Work out the finished part from the listing and answer in its coordinate system (mm). A direction names the side the tool comes from. Round coordinates to 2 decimals unless told otherwise and drop trailing zeros. Order: outer loops, then holes, each group sorted by start corner. A loop starts at its lowest first (then second) coordinate and runs counter-clockwise, first axis right, second up. Notation, with made-up numbers: (13.5, 86.5) - (29.5, 86.5) arc R13 ccw to (29.5, 100.5) - close; hole circle Ø7 at (-35, 75.25). An arc over 180 degrees is marked (long way). Put each result on its own line as item: value.
Autodesk Inventor part; units mm, degrees
ref_plane "YZ Plane" through (0, 0, 0) normal (1, 0, 0) x (0, 1, 0)
ref_plane "XZ Plane" through (0, 0, 0) normal (0, 1, 0) x (-1, 0, 0)
ref_plane "XY Plane" through (0, 0, 0) normal (0, 0, 1) x (1, 0, 0)
sketch "Esboço1" plane through (0, 0, 0) normal (0, 0, 1) x (1, 0, 0)
  line L0 (0, 0) -> (10, 0)
  line L1 (0, 51.1555) -> (0, 0)
  line L2 (2, 35) -> (2, 18.8445)
  line L3 (2, 35) -> (2, 51.1555)
  arc A0 (2, 18.8445) -> (10, 0) centre (66.25, 35) ccw
  line L4 (2, 51.1555) -> (0, 51.1555)
extrude "Extrusão1" add sketch "Esboço1" along normal blind 80
sketch "Esboço2" plane through (0, 0, 80) normal (0, 0, 1) x (1, 0, 0)
  line L0 (0, 0) -> (10, 0)
  line L1 (0, 0) -> (-3, 0)
  line L2 (-5, 2) -> (-5, 2.6)
  line L3 (-5, 2.6) -> (0, 2.6)
  line L4 (-3, 0) -> (-5, 2)
  line L5 (0, 51.1555) -> (0, 0)
  line L6 (0, 2.6) -> (0, 0)
  point P0 (-5, 0)
  dimension "d5" = 5
  dimension "d6" = 2.6
  dimension "d7" = 2
  dimension "d8" = 2
extrude "Extrusão2" add sketch "Esboço2" against normal blind 80
sketch "Esboço3" plane through (2, 18.8445, 0) normal (1, 0, 0) x (0, 0, -1)
  line L0 (0, 0) -> (-80, 0)
  line L1 (-2.5, 11.7555) -> (-77.5, 11.7555)
  line L2 (-2.5, 11.7555) -> (-2.5, -13.7445)
  line L3 (-77.5, -13.7445) -> (-2.5, -13.7445)
  line L4 (-77.5, 11.7555) -> (-77.5, -13.7445)
  line L5 (-77.5, 11.7555) -> (-40, 0) construction
  line L6 (-40, 0) -> (-2.5, 11.7555) construction
  circle A0 centre (-58.75, 5.8777) radius 1.4
  circle A1 centre (-21.25, 5.8777) radius 1.4
  point P0 (0, -18.8445)
  dimension "d11" = 2.8
  dimension "d12" = 2.8
extrude "Extrusão3" cut sketch "Esboço3" against normal blind 80 contours A0 | A1
properties part number "Rampa"
1) Straight lines are drawn through the part: L1, parallel to Y at x = 1.25, z = 21.25; L2, parallel to X at y = 27.5, z = 24.5; L3, parallel to Y at x = -2.75, z = 36.5. For each, find the intervals that lie inside material, in ascending order. Write a range as from..to.
Findings below:
L1: y = 0..23.32, 26.12..51.16
L2: x = 0..2
L3: y = 0..2.6
2) A cutting plane is placed at C-C on y = 47. Write down the section's boundary in (x, z).
Findings below:
outline: (0, 0) - (2, 0) - (2, 80) - (0, 80) - close
3) A cutting plane is placed at D-D on x = -2. Write down the section's boundary in (y, z), then the cut area to 3 significant figures.
Findings below:
outline: (0, 0) - (2.6, 0) - (2.6, 80) - (0, 80) - close
area: 208 mm2
4) For a pull along Z with two mould halves and no side action, classify faces 1 (the flat face through (-4, 1, 41)), 2 (the flat face through (2, 18, 0)), 3 (the cylindrical face through (1.014, 25.903, 20.497)) as pulls with the +Z half, pulls with the -Z half, needs draft (parallel to the pull), parting line crosses it, or undercut.
Findings below:
face 1: needs draft
face 2: pulls with the -Z half
face 3: undercut
5) Given pin 1 Ø1.5 at (x, z) = (-1.5, 29) entering from +Y; pin 2 Ø4 at (y, z) = (29, 28.5) entering from -X; pin 3 Ø6 at (y, z) = (13, 49.5) entering from +X, each flat-ended and moving along its own axis, determine where each tip first touches the part or whether it passes through.
Findings below:
pin 1: stops at y = 2.6
pin 2: stops at x = 0
pin 3: stops at x = 4.9
6) A cutting plane is placed at B-B on z = 47. Write down the section's boundary in (x, y).
Findings below:
outline: (-5, 2) - (-3, 0) - (10, 0) arc R66.25 cw to (2, 18.84) - (2, 51.16) - (0, 51.16) - (0, 2.6) - (-5, 2.6) - close
7) A cutting plane is placed at A-A on z = 21.25. Write down the section's boundary in (x, y), then the cut area to 3 significant figures.
Findings below:
outline: (-5, 2) - (-3, 0) - (10, 0) arc R66.25 cw to (2, 18.84) - (2, 23.32) - (0, 23.32) - (0, 2.6) - (-5, 2.6) - close; (0, 26.12) - (2, 26.12) - (2, 51.16) - (0, 51.16) - close
area: 172 mm2
8) For faces 4 (the flat face through (2, 35, 39)), 5 (the flat face through (2, 18, 80)), 6 (the flat face through (-3, 2.6, 41)), determine the directions among +Z, -Z, +X, -X, +Y, -Y from which every point of the face is accessible in a straight line to the end or side of a thin tool.
Findings below:
face 4: +Z, -Z, +X, +Y
face 5: +Z, +X, -X, +Y, -Y
face 6: +Z, -Z, -X, +Y
